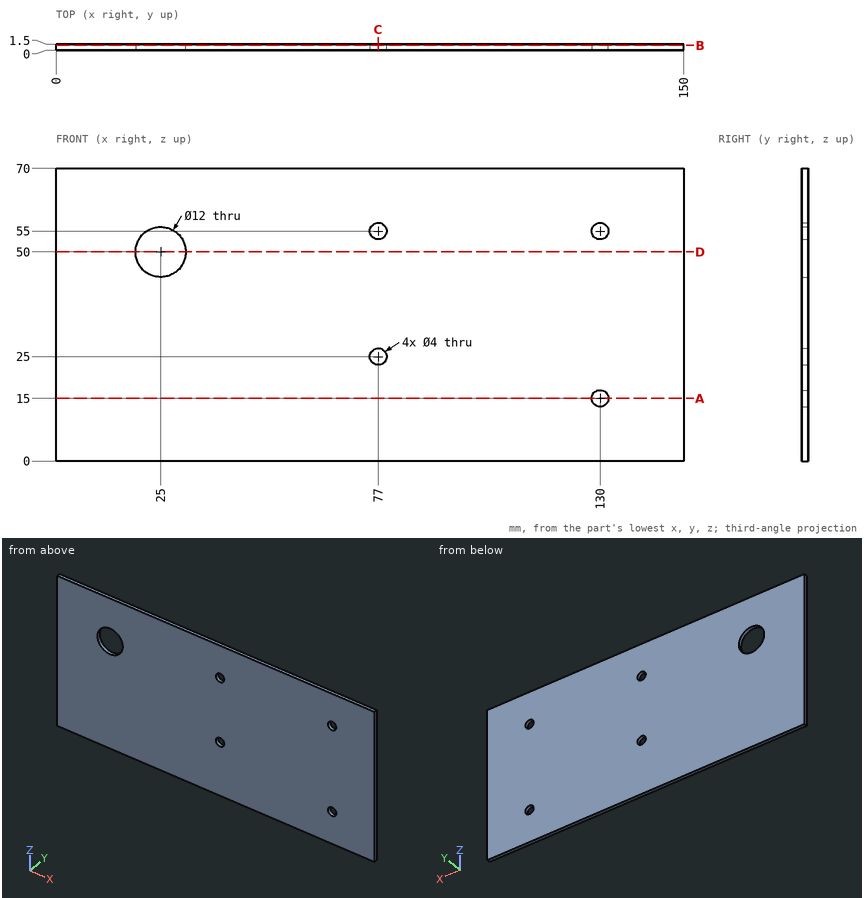
Geometry check sheet. Reference: drawing and pictorial views, mm from the part's lowest x, y, z. Round coordinates to 2 decimals unless told otherwise and drop trailing zeros. Loops run counter-clockwise (first coordinate to the right, second up) from the corner with the lowest first, then second, coordinate; pieces in that order, holes last. Notation, with made-up numbers: (58, 37) - (95, 37) arc R28 ccw to (95, 68) - close; hole circle Ø5 at (-9.75, 67.5). An arc over 180 degrees is marked (long way). Write item = value, one per line. Start each with the question number.
Q1. Section check C-C (x = 77). Record the boundary of the cut face in (y, z), plus the area to 3 significant figures.
Q2. Section check A-A (z = 15). Record the boundary of the cut face in (x, y).
Q3. Section check B-B (y = 1.15). Record the boundary of the cut face in (x, z), plus the area to 3 significant figures.
Q4. Thickness scan on L1, parallel to Z at x = 130, y = 0.6; L2, parallel to Z at x = 77, y = 0.8; L3, parallel to X at y = 0.55, z = 54. Record the ranges inside material, lowest first.
Q5. Section check D-D (z = 50). Record the boundary of the cut face in (x, y), plus the area to 3 significant figures.
Derived:
q1.outline = (0, 0) - (1.5, 0) - (1.5, 23) - (0, 23) - close; (0, 27) - (1.5, 27) - (1.5, 53) - (0, 53) - close; (0, 57) - (1.5, 57) - (1.5, 70) - (0, 70) - close
q1.area = 93.0 mm^2
q2.outline = (0, 0) - (128, 0) - (128, 1.5) - (0, 1.5) - close; (132, 0) - (150, 0) - (150, 1.5) - (132, 1.5) - close
q3.outline = (0, 0) - (150, 0) - (150, 70) - (0, 70) - close; hole circle Ø12 at (25, 50); hole circle Ø4 at (77, 25); hole circle Ø4 at (77, 55); hole circle Ø4 at (130, 15); hole circle Ø4 at (130, 55)
q3.area = 10,300 mm^2
q4.L1 = 0 to 13, 17 to 53, 57 to 70
q4.L2 = 0 to 23, 27 to 53, 57 to 70
q4.L3 = 0 to 20.53, 29.47 to 75.27, 78.73 to 128.27, 131.73 to 150
q5.outline = (0, 0) - (19, 0) - (19, 1.5) - (0, 1.5) - close; (31, 0) - (150, 0) - (150, 1.5) - (31, 1.5) - close
q5.area = 207 mm^2
